Here's how the part is built. I have some questions about the finished solid (model axes, mm). Face numbers are marked on the shaded views. A direction names the side the tool comes from. Coordinates: 2 decimals unless noted, no trailing zeros. Order: outer loops, then holes, each group sorted by start corner. A loop starts at its lowest first (then second) coordinate and runs counter-clockwise, first axis right, second up. Notation, with made-up numbers: (-4.5, -21) - (24.5, -21) arc R3 ccw to (24.5, -17) - close; hole circle Ø6 at (57.5, -29). An arc over 180 degrees is marked (long way). Answer in a Markdown table with one row per item. Add a question column.
Item 1: Will these pins go through, and if not, where does the flat tip stop? pin 1 Ø5.5 at (x, z) = (-1.5, -0.5) entering from -Y; pin 2 Ø6 at (x, z) = (-15, -6.5) entering from -Y; pin 3 Ø4 at (x, z) = (13, -23) entering from +Y; pin 4 Ø5 at (y, z) = (3, 11.5) entering from -X.
Item 2: On a 3-axis mill with a long thin cutter (end or side, diameter ignored), from which of +Z, -Z, +X, -X, +Y, -Y can I reach the whole of each face in a straight line? I mean the marked faces 4 and 5. Say none if no direction works.
Item 3: I want a section at A-A (y = 5). Please give me the cut outline in (x, z).
Item 4: If I drill on line 1 along Z through (x, y) = (0, 0.2); line 2 along Y through (x, z) = (-9, 23.5), over which ranges is the centre line in solid material (lowest first)? Write a range as from..to.
Item 5: I want a section at D-D (x = 23). Please give me the cut outline in (y, z).
Item 6: Thinking about a two-plate mould opening in Z: for the marked faces 1, 2 and 3, which applies, +Z half, -Z half, draft (parallel to the pull), parting line (faces both ways), or undercut?
Item 7: I want a section at B-B (z = 0). Count the separate pieces of the cut face and the enclosed holes in it, plus the area to 4 significant figures.
```python
from build123d import *

# Parameters (mm, degrees)
SKETCH1_R           = 31
SKETCH1_R_2         = 25
BOSS_EXTRUDE1_DEPTH = 1.2
SKETCH2_R           = 26.2
SKETCH2_R_2         = 25
BOSS_EXTRUDE2_DEPTH = 6.5
SKETCH3_R           = 26.2
BOSS_EXTRUDE3_DEPTH = 1.5
CUT_EXTRUDE2_DEPTH  = 5
CUT_EXTRUDE3_START  = -0.5
SKETCH7_R           = 25.6
SKETCH7_R_2         = 25
CUT_EXTRUDE3_DEPTH  = 3
FILLET1_R           = 0.75
SKETCH8_R           = 3.5
SKETCH8_R_2         = 2
BOSS_EXTRUDE4_DEPTH = 3.5


with BuildPart() as part:
    # Sketch1 → Boss-Extrude1 (new body)
    with BuildSketch(Plane(origin=(0, 0, 0), x_dir=(1, 0, 0), z_dir=(0, 1, 0))):
        Circle(SKETCH1_R)
        Circle(SKETCH1_R_2, mode=Mode.SUBTRACT)
    extrude(amount=BOSS_EXTRUDE1_DEPTH)

    # Sketch2 → Boss-Extrude2 (add)
    with BuildSketch(Plane(origin=(0, 1.2, 0), x_dir=(1, 0, 0), z_dir=(0, 1, 0))):
        Circle(SKETCH2_R)
        Circle(SKETCH2_R_2, mode=Mode.SUBTRACT)
    extrude(amount=BOSS_EXTRUDE2_DEPTH)

    # Sketch3 → Boss-Extrude3 (add)
    with BuildSketch(Plane(origin=(0, 7.7, 0), x_dir=(1, 0, 0), z_dir=(0, 1, 0))):
        Circle(SKETCH3_R)
    extrude(amount=BOSS_EXTRUDE3_DEPTH)

    # Sketch5 → Cut-Extrude2 (cut)
    with BuildSketch(Plane(origin=(0, 9.2, 0), x_dir=(1, 0, 0), z_dir=(0, 1, 0))):
        with BuildLine():
            Line((20.525667656, 16.283026969), (19.671249118, 15.428608431))
            ThreePointArc((19.671249118, 15.428608431), (25, 0), (19.671249118, -15.428608431))
            Line((19.671249118, -15.428608431), (20.525667656, -16.283026969))
            ThreePointArc((20.525667656, -16.283026969), (26.2, 0), (20.525667656, 16.283026969))
        make_face()
        with BuildLine():
            Line((16.283026969, -20.525667656), (15.428608431, -19.671249118))
            ThreePointArc((15.428608431, -19.671249118), (0, -25), (-15.428608431, -19.671249118))
            Line((-15.428608431, -19.671249118), (-16.283026969, -20.525667656))
            ThreePointArc((-16.283026969, -20.525667656), (0, -26.2), (16.283026969, -20.525667656))
        make_face()
        with BuildLine():
            Line((-19.671249118, -15.428608431), (-20.525667656, -16.283026969))
            ThreePointArc((-20.525667656, -16.283026969), (-26.2, 0), (-20.525667656, 16.283026969))
            Line((-20.525667656, 16.283026969), (-19.671249118, 15.428608431))
            ThreePointArc((-19.671249118, 15.428608431), (-25, 0), (-19.671249118, -15.428608431))
        make_face()
    extrude(amount=-CUT_EXTRUDE2_DEPTH, mode=Mode.SUBTRACT)

    # Sketch7 → Cut-Extrude3 (cut)
    with BuildSketch(Plane.XZ.offset(CUT_EXTRUDE3_START)):
        Circle(SKETCH7_R)
        Circle(SKETCH7_R_2, mode=Mode.SUBTRACT)
    extrude(amount=-CUT_EXTRUDE3_DEPTH, mode=Mode.SUBTRACT)

    # Fillet1
    fillet1_edges = [part.edges().sort_by_distance(p)[0] for p in [
        (18.526197667, 9.2, 18.526197667),
        (0, 9.2, -26.2),
        (-18.526197667, 9.2, 18.526197667),
    ]]
    fillet(fillet1_edges, radius=FILLET1_R)

    # Sketch8 → Boss-Extrude4 (add)
    with BuildSketch(Plane.XZ.offset(-7.7)):
        Circle(SKETCH8_R)
        Circle(SKETCH8_R_2, mode=Mode.SUBTRACT)
    extrude(amount=BOSS_EXTRUDE4_DEPTH)


solid = part.part
```
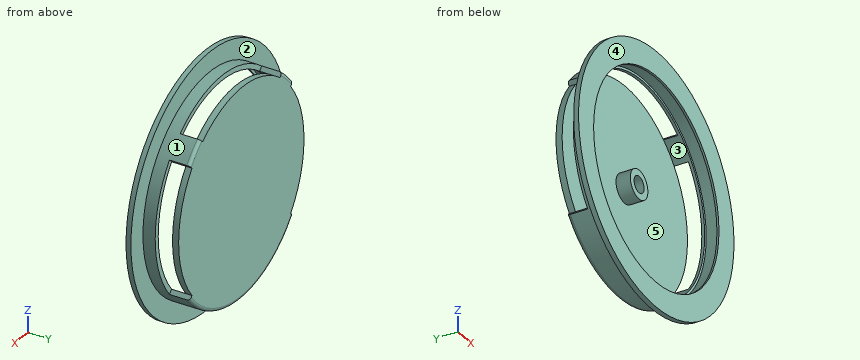
Values follow:
| question | item | result |
|---|---|---|
| 1 | pin 1 | stops at y = 4.2 |
| 1 | pin 2 | stops at y = 7.7 |
| 1 | pin 3 | stops at y = 9.2 |
| 1 | pin 4 | stops at x = -29.42 |
| 2 | face 4 | +Z, -Z, +X, -X, -Y |
| 2 | face 5 | -Y |
| 3 | outline | (-20.53, -16.28) arc R26.2 ccw to (20.53, -16.28) - (19.67, -15.43) arc R25 cw to (-19.67, -15.43) - close; (-20.53, 16.28) - (-19.67, 15.43) arc R25 cw to (-15.43, 19.67) - (-16.28, 20.53) arc R26.2 ccw to start; circle Ø7 at (0, 0); (15.43, 19.67) arc R25 cw to (19.67, 15.43) - (20.53, 16.28) arc R26.2 ccw to (16.28, 20.53) - close; hole circle Ø4 at (0, 0) |
| 4 | line 1 | z = -31..-25, 25..31 |
| 4 | line 2 | y = 0..0.5, 3.5..4.2 |
| 5 | outline | (0, -20.78) - (1.2, -20.78) - (1.2, -12.55) - (4.2, -12.55) - (4.2, -9.8) - (3.5, -9.8) - (3.5, -11.24) - (0.5, -11.24) - (0.5, -9.8) - (0, -9.8) - close; (0, 9.8) - (0.5, 9.8) - (0.5, 11.24) - (3.5, 11.24) - (3.5, 9.8) - (4.2, 9.8) - (4.2, 12.55) - (1.2, 12.55) - (1.2, 20.78) - (0, 20.78) - close; (7.7, -9.8) - (9.2, -9.8) - (9.2, 9.8) - (7.7, 9.8) - close |
| 6 | face 1 | parting line |
| 6 | face 2 | draft |
| 6 | face 3 | undercut |
| 7 | separate pieces | 3 |
| 7 | enclosed holes | 0 |
| 7 | area | 103.5 mm^2 |
